Source: CAD feature listing. Evaluate the final solid. Frame: model axes, mm. A direction names the side the tool comes from. Round coordinates to 2 decimals unless told otherwise and drop trailing zeros. Loops run counter-clockwise (first coordinate to the right, second up) from the corner with the lowest first, then second, coordinate; pieces in that order, holes last. Notation, with made-up numbers: (-35, -1.5) - (15, -1.5) arc R23 ccw to (15, 30.5) - close; hole circle Ø4 at (75.5, 42.25). An arc over 180 degrees is marked (long way). One line per question, with ' | ' between items.
from build123d import *

# Parameters (mm, degrees)
ESBO_O1_R                = 13.5
ESBO_O1_R_2              = 5.5
RESSALTO_EXTRUS_O1_DEPTH = 3
ESBO_O2_R                = 7.5
ESBO_O2_R_2              = 5.5
RESSALTO_EXTRUS_O2_DEPTH = 51
ESBO_O3_R                = 13.5
ESBO_O3_R_2              = 5.5
RESSALTO_EXTRUS_O3_DEPTH = 3


with BuildPart() as part:
    # Esboço1 → Ressalto-extrusão1 (new body)
    with BuildSketch(Plane.XY):
        Circle(ESBO_O1_R)
        Circle(ESBO_O1_R_2, mode=Mode.SUBTRACT)
    extrude(amount=RESSALTO_EXTRUS_O1_DEPTH)

    # Esboço2 → Ressalto-extrusão2 (add)
    with BuildSketch(Plane.XY.offset(3)):
        Circle(ESBO_O2_R)
        Circle(ESBO_O2_R_2, mode=Mode.SUBTRACT)
    extrude(amount=RESSALTO_EXTRUS_O2_DEPTH)

    # Esboço3 → Ressalto-extrusão3 (add)
    with BuildSketch(Plane.XY.offset(54)):
        Circle(ESBO_O3_R)
        Circle(ESBO_O3_R_2, mode=Mode.SUBTRACT)
    extrude(amount=RESSALTO_EXTRUS_O3_DEPTH)


solid = part.part
1. Section query C-C, the plane x = 11. Return loops of the section in (y, z).
Worked out:
outline: (-7.83, 0) - (7.83, 0) - (7.83, 3) - (-7.83, 3) - close; (-7.83, 54) - (7.83, 54) - (7.83, 57) - (-7.83, 57) - close
2. Section query D-D, the plane z = 39. Return loops of the section in (x, y).
Worked out:
outline: circle Ø15 at (0, 0); hole circle Ø11 at (0, 0)
3. Access query for faces 4 (the flat face through (6, -6, 54)), 5 (the cylindrical face through (-2.93, -13.18, 1.48)). Directions: +Z, -Z, +X, -X, +Y, -Y. A direction counts if a zero-diameter tool reaches every point of the face in a straight line with its end or side. Return the directions, or none.
Worked out:
face 4: none | face 5: +Z, -Z
4. Mould query, pull axis Y, two halves, no side actions, for faces 1 (the flat face through (6, 0, 0)), 2 (the cylindrical face through (-1.19, -5.37, 28.1)), 3 (the cylindrical face through (-2.93, -13.18, 55.48)). Classes: released by +Y, released by -Y, zero draft, split by the parting line, or undercut.
Worked out:
face 1: zero draft | face 2: undercut | face 3: split by the parting line
5. Section query A-A, the plane x = 0. Return loops of the section in (y, z).
Worked out:
outline: (-13.5, 0) - (-5.5, 0) - (-5.5, 57) - (-13.5, 57) - (-13.5, 54) - (-7.5, 54) - (-7.5, 3) - (-13.5, 3) - close; (5.5, 0) - (13.5, 0) - (13.5, 3) - (7.5, 3) - (7.5, 54) - (13.5, 54) - (13.5, 57) - (5.5, 57) - close
6. Contact query for flat-ended pins moving along their axis: P1, Ø6, axis at x = 1.5, z = 32.5, coming from the +Y side; P2, Ø6, axis at y = 6, z = 39, coming from the +X side; P3, Ø2, axis at y = -5, z = 32.5, coming from the +X side. Output: stop coordinate, or through.
Worked out:
P1: stops at y = 7.5 | P2: stops at x = 6.87 | P3: stops at x = 6.34
7. Material intervals for probe 1 along Y at (x, z) = (0, 17.5); probe 2 along Z at (x, y) = (-1.75, 7.5); probe 3 along X at (y, z) = (-2, 24), sorted ascending.
Worked out:
probe 1: y = -7.5 to -5.5, 5.5 to 7.5 | probe 2: z = 0 to 3, 54 to 57 | probe 3: x = -7.23 to -5.12, 5.12 to 7.23
